Input: part model. Units: mm. Frame: model coordinates. A direction names the side the tool comes from. Give positions to 0.01 mm unless a question says otherwise; leave off trailing zeros. Order: outer loops, then holes, each group sorted by start corner. A loop starts at its lowest first (then second) coordinate and runs counter-clockwise, first axis right, second up. Notation, with made-up numbers: (-28.5, 67) - (4.5, 67) arc R20 ccw to (4.5, 89) - close; hole circle Ø2 at (-9.75, 36.25). An arc over 180 degrees is marked (long way). Answer in a Markdown table with one row per item. Add a question column.
from build123d import *

# Parameters (mm, degrees)
SKETCH2_R           = 2.05
SKETCH2_R_2         = 0.700643725
BOSS_EXTRUDE1_DEPTH = 2
SKETCH3_W           = 5.75
SKETCH3_H           = 4
BOSS_EXTRUDE2_DEPTH = 4.5
SKETCH4_R           = 0.65
CUT_EXTRUDE1_DEPTH  = 18.578324987
BOSS_EXTRUDE3_DEPTH = 2


with BuildPart() as part:
    # Sketch2 → Boss-Extrude1 (new body)
    with BuildSketch(Plane(origin=(0, 0, 0), x_dir=(1, 0, 0), z_dir=(0, 1, 0))):
        Polygon((-3.5, -6.76929), (-3.5, -0.98071), (3.5, -0.98071), (3.5, -6.76929), (13.7785, -6.76929), (13.7785, 6.76929), (-13.7785, 6.76929), (-13.7785, -6.76929), align=None)
        with Locations(Location((-8.7785, -1.76929, 0), (0, 0, 270))):
            Circle(SKETCH2_R, mode=Mode.SUBTRACT)
        with Locations(Location((8.9015, -1.76929, 0), (0, 0, 270))):
            Circle(SKETCH2_R, mode=Mode.SUBTRACT)
        with Locations(Location((0.0585, 1.07400228, 0), (0, 0, 270))):
            Circle(SKETCH2_R_2, mode=Mode.SUBTRACT)
    extrude(amount=BOSS_EXTRUDE1_DEPTH)

    # Sketch3 → Boss-Extrude2 (add)
    with BuildSketch(Plane(origin=(0, 2, 0), x_dir=(1, 0, 0), z_dir=(0, 1, 0))):
        with Locations((-5.125, 6.76929)):
            Rectangle(SKETCH3_W, SKETCH3_H)
        with Locations((5.125, 6.76929)):
            Rectangle(SKETCH3_W, SKETCH3_H)
    extrude(amount=BOSS_EXTRUDE2_DEPTH)

    # Sketch4 → Cut-Extrude1 (cut, through all)
    with BuildSketch(Plane(origin=(0, 6.5, 0), x_dir=(1, 0, 0), z_dir=(0, 1, 0))):
        with Locations(Location((-5.94, 7.06929, 0), (0, 0, 270))):
            Circle(SKETCH4_R)
        with Locations(Location((6.06, 7.06929, 0), (0, 0, 270))):
            Circle(SKETCH4_R)
    extrude(amount=-CUT_EXTRUDE1_DEPTH, mode=Mode.SUBTRACT)

    # Sketch5 → Boss-Extrude3 (add)
    with BuildSketch(Plane(origin=(0, 2, 0), x_dir=(1, 0, 0), z_dir=(0, 1, 0))):
        Polygon((-13.7785, 6.76929), (-23.7785, 6.76929), (-23.7785, -16.768919175), (-3.413881725, -16.768919175), (-3.5, -6.76929), (-13.7785, -6.76929), align=None)
        Polygon((3.5, -6.76929), (3.5, -16.768919175), (23.7785, -16.768919175), (23.7785, 6.76929), (13.7785, 6.76929), (13.7785, -6.76929), align=None)
    extrude(amount=-BOSS_EXTRUDE3_DEPTH)


solid = part.part
Q1. Line query: probe 1 along Z at (x, y) = (-5.94, 4.25); probe 2 along X at (y, z) = (6, -7.5); probe 3 along X at (y, z) = (0.75, 7). Output: solid intervals per line, ascending.
Q2. Section D-D, the plane x = -21. Return loops of the section in (y, z), then the cut area to 3 significant figures.
Q3. Contact query for flat-ended pins moving along their axis: P1, Ø3, axis at y = 4.5, z = -7.5, coming from the -X side; P2, Ø0.6, axis at x = -2.5, y = 1, coming from the -Z side; P3, Ø6, axis at x = -18, z = 13, coming from the +Y side; P4, Ø1.6, axis at x = 0.06, z = -1.07, coming from the -Y side. Output: stop coordinate, or through.
Q4. Pull-direction query (X, two-part tool) for faces 1 (the flat face through (2.25, 4, -7)), 2 (the flat face through (-5, 2, -8)), 3 (the flat face through (8, 4, -7)); classes: +X half, -X half, draft (parallel to the pull), parting line (faces both ways), or undercut.
Q5. Access query for faces 4 (the flat face through (-3.5, 1, 4)), 5 (the flat face through (-2.25, 4, -7)), 6 (the flat face through (5, 4, -4.769)), 7 (the flat face through (0, 1, -6.769)), 8 (the flat face through (13, 1, 16.769)). Directions: +Z, -Z, +X, -X, +Y, -Y. A direction counts if a zero-diameter tool reaches every point of the face in a straight line with its end or side. Return the directions, or none.
Q6. Section C-C, the plane z = 0.25. Return loops of the section in (x, y).
Q7. Section B-B, the plane x = -5.94. Return loops of the section in (y, z), then the cut area to 3 significant figures.
Q8. Section A-A, the plane y = 3.5. Return loops of the section in (x, z).
Computed:
| question | item | result |
|---|---|---|
| 1 | probe 1 | z = -8.77 to -7.72, -6.42 to -4.77 |
| 1 | probe 2 | x = -8 to -6.43, -5.45 to -2.25, 2.25 to 5.57, 6.55 to 8 |
| 1 | probe 3 | x = -23.78 to -3.5, 3.5 to 23.78 |
| 2 | outline | (0, -6.77) - (2, -6.77) - (2, 16.77) - (0, 16.77) - close |
| 2 | area | 47.1 mm^2 |
| 3 | P1 | stops at x = -8 |
| 3 | P2 | stops at z = -6.77 |
| 3 | P3 | stops at y = 2 |
| 3 | P4 | stops at y = 0 |
| 4 | face 1 | undercut |
| 4 | face 2 | draft |
| 4 | face 3 | +X half |
| 5 | face 4 | +Y, -Y |
| 5 | face 5 | +Z, -Z, +Y |
| 5 | face 6 | +Z, +X, -X, +Y |
| 5 | face 7 | -Z, +X, -X, -Y |
| 5 | face 8 | +Z, +X, -X, +Y, -Y |
| 6 | outline | (-23.78, 0) - (-10.15, 0) - (-10.15, 2) - (-23.78, 2) - close; (-7.4, 0) - (7.53, 0) - (7.53, 2) - (-7.4, 2) - close; (10.28, 0) - (23.78, 0) - (23.78, 2) - (10.28, 2) - close |
| 7 | outline | (0, -6.42) - (6.5, -6.42) - (6.5, -4.77) - (2, -4.77) - (2, 16.77) - (0, 16.77) - close; (2, -8.77) - (6.5, -8.77) - (6.5, -7.72) - (2, -7.72) - close |
| 7 | area | 58.5 mm^2 |
| 8 | outline | (-8, -8.77) - (-2.25, -8.77) - (-2.25, -4.77) - (-8, -4.77) - close; (2.25, -8.77) - (8, -8.77) - (8, -4.77) - (2.25, -4.77) - close; hole circle Ø1.3 at (-5.94, -7.07); hole circle Ø1.3 at (6.06, -7.07) |
